Read the model definition and answer for the solid it produces. Units are mm, in the model's axes. Face numbers are marked on the shaded views. A direction names the side the tool comes from. Coordinates: 2 decimals unless noted, no trailing zeros. Order: outer loops, then holes, each group sorted by start corner. A loop starts at its lowest first (then second) coordinate and runs counter-clockwise, first axis right, second up. Notation, with made-up numbers: (47, 3) - (62, 3) arc R10 ccw to (62, 20) - close; hole circle Ø3 at (-2, 11.5). An arc over 180 degrees is marked (long way). Write item = value, one per line.
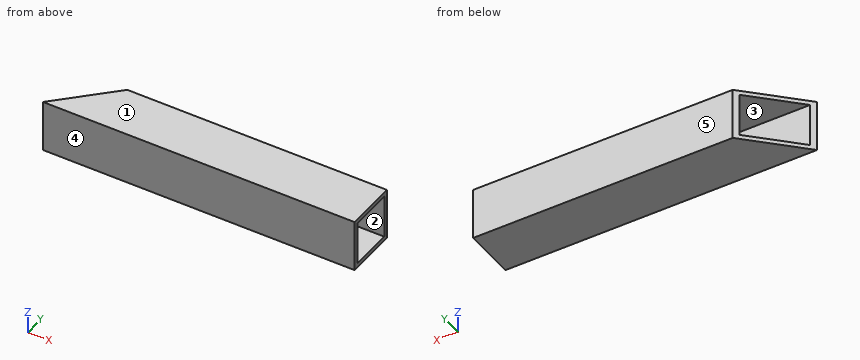
from build123d import *

# Parameters (mm, degrees)
SKETCH1_W                              = 25.4
SKETCH1_H                              = 25.4
SKETCH1_W_2                            = 21.1836
SKETCH1_H_2                            = 21.1836
AL_TUBE_SQUARE_1_SQ_X_083_WALL_1_DEPTH = 152.4
CORTAR_EXTRUIR1_DEPTH                  = 58.928


with BuildPart() as part:
    # Sketch1 → Al tube (square) 1 SQ X .083 WALL(1) (new body)
    with BuildSketch(Plane.YZ):
        Rectangle(SKETCH1_W, SKETCH1_H)
        Rectangle(SKETCH1_W_2, SKETCH1_H_2, mode=Mode.SUBTRACT)
    extrude(amount=AL_TUBE_SQUARE_1_SQ_X_083_WALL_1_DEPTH)

    # Croquis3 → Cortar-Extruir1 (cut)
    with BuildSketch(Plane.XY.offset(12.7)):
        Polygon((0, -12.7), (25.4, 12.7), (0, 12.7), align=None)
    extrude(amount=-CORTAR_EXTRUIR1_DEPTH, mode=Mode.SUBTRACT)


solid = part.part
1) The part is cut by section D-D (x = 11). Determine the outline of the cut face in (y, z), and give its area (3 significant figures).
Returned:
outline = (-12.7, -12.7) - (-1.7, -12.7) - (-1.7, -10.59) - (-10.59, -10.59) - (-10.59, 10.59) - (-1.7, 10.59) - (-1.7, 12.7) - (-12.7, 12.7) - close
area = 91.0 mm^2
2) Determine the mould class of the marked faces 3, 4 and 5 for opening direction Y: pulls with the +Y half, pulls with the -Y half, needs draft (parallel to the pull), parting line crosses it, or undercut.
Returned:
face_3 = undercut
face_4 = pulls with the -Y half
face_5 = pulls with the +Y half
3) Straight lines are drawn through the part: line 1 along Z through (x, y) = (64.5, 1.25); line 2 along Y through (x, z) = (8.5, 3). For each, find the intervals that lie inside material, in ascending order. Write a range as from..to.
Returned:
line_1 = -12.7..-10.59, 10.59..12.7
line_2 = -12.7..-10.59
4) The part is cut by section A-A (y = -8.75). Determine the outline of the cut face in (x, z).
Returned:
outline = (3.95, -12.7) - (152.4, -12.7) - (152.4, -10.59) - (3.95, -10.59) - close; (3.95, 10.59) - (152.4, 10.59) - (152.4, 12.7) - (3.95, 12.7) - close
5) For the marked faces 1 and 2, determine the directions among +Z, -Z, +X, -X, +Y, -Y from which every point of the face is accessible in a straight line to the end or side of a thin tool.
Returned:
face_1 = +Z, +X, -X, +Y, -Y
face_2 = +X, -X
6) The part is cut by section C-C (z = 7). Determine the outline of the cut face in (x, y), and give its area (3 significant figures).
Returned:
outline = (0, -12.7) - (152.4, -12.7) - (152.4, -10.59) - (2.11, -10.59) - close; (23.29, 10.59) - (152.4, 10.59) - (152.4, 12.7) - (25.4, 12.7) - close
area = 589 mm^2
7) The part is cut by section B-B (x = 80.5). Determine the outline of the cut face in (y, z), and give its area (3 significant figures).
Returned:
outline = (-12.7, -12.7) - (12.7, -12.7) - (12.7, 12.7) - (-12.7, 12.7) - close; hole (-10.59, -10.59) - (10.59, -10.59) - (10.59, 10.59) - (-10.59, 10.59) - close
area = 196 mm^2
